For this review, take the finished solid that the model builds, in its own axes (mm). A direction names the side the tool comes from. Round coordinates to 2 decimals unless told otherwise and drop trailing zeros. Order: outer loops, then holes, each group sorted by start corner. A loop starts at its lowest first (then second) coordinate and runs counter-clockwise, first axis right, second up. Notation, with made-up numbers: (-29, 71) - (24, 71) arc R33 ccw to (24, 99) - close; hole circle Ø2 at (61.25, 28.5). An arc over 180 degrees is marked (long way). One line per item, written item: value.
```python
from build123d import *

# Parameters (mm, degrees)
SKETCH1_R           = 19
SKETCH1_R_2         = 17.2
BOSS_EXTRUDE1_DEPTH = 33
SKETCH1_3_R         = 11.5
SKETCH1_3_R_2       = 9.7
BOSS_EXTRUDE2_DEPTH = 43
SKETCH2_R           = 17.2
BOSS_EXTRUDE3_DEPTH = 3
BOSS_EXTRUDE4_DEPTH = 2.4
BOSS_EXTRUDE5_DEPTH = 5
SKETCH5_R           = 1.5
CUT_EXTRUDE1_DEPTH  = 44


with BuildPart() as part:
    # Sketch1 → Boss-Extrude1 (new body)
    with BuildSketch(Plane(origin=(0, 0, 0), x_dir=(1, 0, 0), z_dir=(0, 1, 0))):
        Circle(SKETCH1_R)
        Circle(SKETCH1_R_2, mode=Mode.SUBTRACT)
    extrude(amount=BOSS_EXTRUDE1_DEPTH)



with BuildPart() as body_2:
    # Sketch1_3 → Boss-Extrude2 (new body)
    with BuildSketch(Plane(origin=(0, 0, 0), x_dir=(1, 0, 0), z_dir=(0, 1, 0))):
        Circle(SKETCH1_3_R)
        Circle(SKETCH1_3_R_2, mode=Mode.SUBTRACT)
    extrude(amount=BOSS_EXTRUDE2_DEPTH)


with BuildPart() as part_1:
    add(part.part)

    add(body_2.part)  # Boss-Extrude3 merges body 2
    # Sketch2 → Boss-Extrude3 (add)
    with BuildSketch(Plane(origin=(0, 10, 0), x_dir=(-1, 0, 0), z_dir=(0, -1, 0))):
        Circle(SKETCH2_R)
    extrude(amount=-BOSS_EXTRUDE3_DEPTH)

    # Sketch3 → Boss-Extrude4 (add)
    with BuildSketch(Plane.XZ):
        with BuildLine():
            Line((-14.921917905, -11.7616481), (-5.15253427, -5.060203124))
            Line((-5.15253427, -5.060203124), (-3.565454801, -6.280270465))
            Line((-3.565454801, -6.280270465), (-7.530041661, -17.444152963))
            ThreePointArc((-7.530041661, -17.444152963), (-11.579954122, -15.063354956), (-14.921917905, -11.7616481))
        make_face()
    extrude(amount=-BOSS_EXTRUDE4_DEPTH)

    # Sketch4 → Boss-Extrude5 (add)
    with BuildSketch(Plane.XZ):
        with BuildLine():
            Line((-5.5, 16.296932227), (-5.5, 10.099504938))
            ThreePointArc((-5.5, 10.099504938), (0, 11.5), (5.5, 10.099504938))
            Line((5.5, 10.099504938), (5.5, 16.296932227))
            ThreePointArc((5.5, 16.296932227), (0, 17.2), (-5.5, 16.296932227))
        make_face()
        with BuildLine():
            Line((-5.5, 18.186533479), (-5.5, 16.296932227))
            ThreePointArc((-5.5, 16.296932227), (0, 17.2), (5.5, 16.296932227))
            Line((5.5, 16.296932227), (5.5, 18.186533479))
            ThreePointArc((5.5, 18.186533479), (0, 19), (-5.5, 18.186533479))
        make_face()
        with BuildLine():
            Line((-5.5, 48), (-5.5, 18.186533479))
            ThreePointArc((-5.5, 18.186533479), (0, 19), (5.5, 18.186533479))
            Line((5.5, 18.186533479), (5.5, 48))
            Line((5.5, 48), (-5.5, 48))
        make_face()
        with BuildLine():
            Line((-5.5, 10.099504938), (-5.5, 7.989993742))
            ThreePointArc((-5.5, 7.989993742), (0, 9.7), (5.5, 7.989993742))
            Line((5.5, 7.989993742), (5.5, 10.099504938))
            ThreePointArc((5.5, 10.099504938), (0, 11.5), (-5.5, 10.099504938))
        make_face()
    extrude(amount=-BOSS_EXTRUDE5_DEPTH)

    # Sketch5 → Cut-Extrude1 (cut, through all)
    with BuildSketch(Plane.XZ):
        with Locations((0, 44)):
            Circle(SKETCH5_R)
    extrude(amount=-CUT_EXTRUDE1_DEPTH, mode=Mode.SUBTRACT)


solid = part_1.part
```
Item 1: Take a section at C-C (y = 14.5). Write out the cut boundary in (x, z), plus the area to 3 significant figures.
Returned:
outline: circle Ø38 at (0, 0); circle Ø23 at (0, 0); hole circle Ø34.4 at (0, 0); hole circle Ø19.4 at (0, 0)
area: 325 mm^2
Item 2: Take a section at B-B (z = 44). Write out the cut boundary in (x, y).
Returned:
outline: (-5.5, 0) - (-1.5, 0) - (-1.5, 5) - (-5.5, 5) - close; (1.5, 0) - (5.5, 0) - (5.5, 5) - (1.5, 5) - close
Item 3: Take a section at D-D (z = 0). Write out the cut boundary in (x, y), plus the area to 3 significant figures.
Returned:
outline: (-19, 0) - (-17.2, 0) - (-17.2, 10) - (-11.5, 10) - (-11.5, 0) - (-9.7, 0) - (-9.7, 10) - (9.7, 10) - (9.7, 0) - (11.5, 0) - (11.5, 10) - (17.2, 10) - (17.2, 0) - (19, 0) - (19, 33) - (17.2, 33) - (17.2, 13) - (11.5, 13) - (11.5, 43) - (9.7, 43) - (9.7, 13) - (-9.7, 13) - (-9.7, 43) - (-11.5, 43) - (-11.5, 13) - (-17.2, 13) - (-17.2, 33) - (-19, 33) - close
area: 366 mm^2
Item 4: Machinability: for faces 4 (the cylindrical face through (-1.5, 4.9, -11.4)), 5 (the flat face through (5.5, 2, 13)), 6 (the cylindrical face through (-17.183, 22.86, -0.756)), which of the approach directions +Z, -Z, +X, -X, +Y, -Y give a long, thin tool a straight path to every point of the face, cutting with its end or side? Answer none if there is none.
Returned:
face 4: none
face 5: -Y
face 6: +Y
Item 5: Take a section at A-A (x = 0). Count the separate pieces of the cut face and the enclosed holes in it, plus the area to 4 significant figures.
Returned:
separate pieces: 2
enclosed holes: 1
area: 524.5 mm^2
Item 6: Wall thickness on line 1 (Z direction, x = 0, y = 2.75); line 2 (Z direction, x = 0, y = 20.5): over which ranges is each line inside the solid? List them lowest first.
Returned:
line 1: -19 to -17.2, -11.5 to -9.7, 9.7 to 42.5, 45.5 to 48
line 2: -19 to -17.2, -11.5 to -9.7, 9.7 to 11.5, 17.2 to 19
Item 7: The part is to be moulded in two halves that separate along Z. For faces 1 (the flat face through (-6, 43, 8)), 2 (the cylindrical face through (10.214, 16.269, -16.021)), 3 (the cylindrical face through (-1.5, 27.8, -11.4)), say which applies: +Z half, -Z half, draft (parallel to the pull), parting line (faces both ways), or undercut.
Returned:
face 1: draft
face 2: parting line
face 3: undercut
Item 8: For P1, Ø6, axis at x = -6, z = 13, coming from the -Y side; P2, Ø8, axis at y = 25.5, z = -4.5, coming from the +X side; P3, Ø5.5, axis at x = 1.5, z = 15, coming from the +Y side; P4, Ø4, axis at y = 3, z = 12, coming from the -X side, all flat-tipped, find the tip position at first contact; note any pin that passes through.
Returned:
P1: y = 0
P2: x = 18.99
P3: y = 33
P4: x = -16.16
